Part print with two shaded views. Sizes in mm from the minimum x, y, z corner. Coordinates: 2 decimals unless noted, no trailing zeros. Order: outer loops, then holes, each group sorted by start corner. A loop starts at its lowest first (then second) coordinate and runs counter-clockwise, first axis right, second up. Notation, with made-up numbers: (-1, -37) - (54, -37) arc R17 ccw to (54, -21) - close; hole circle Ø3 at (56.25, 2.25). An arc over 180 degrees is marked (long way). Write each question's results on one line, items separated by ' | '. Start each with the question number.
Q1. Wall check: probe 1 along X at (y, z) = (51.5, 2.55) (1 decimal); probe 2 along Y at (x, z) = (7, 1.6); probe 3 along Y at (x, z) = (6, 2.4) (1 decimal). Give the ranges that are in metal, low to high.
Q2. Pin check, flat tips, straight feed: P1, Ø8, axis at x = 47, y = 39.5, coming from the -Z side; P2, Ø1.5, axis at y = 34.5, z = 2, coming from the +X side. Stop position of each tip, or through.
Q3. Band-saw the part on C-C, the plane x = 44.5. Write the cut outline in (y, z) (1 decimal).
Q4. Band-saw the part on A-A, the plane z = 1.6. Count the separate pieces of the cut face and the enclosed holes in it, then the cut area to 3 significant figures.
Q5. Band-saw the part on D-D, the plane y = 35.5. Write the cut outline in (x, z) (1 decimal), then the cut area to 3 significant figures.
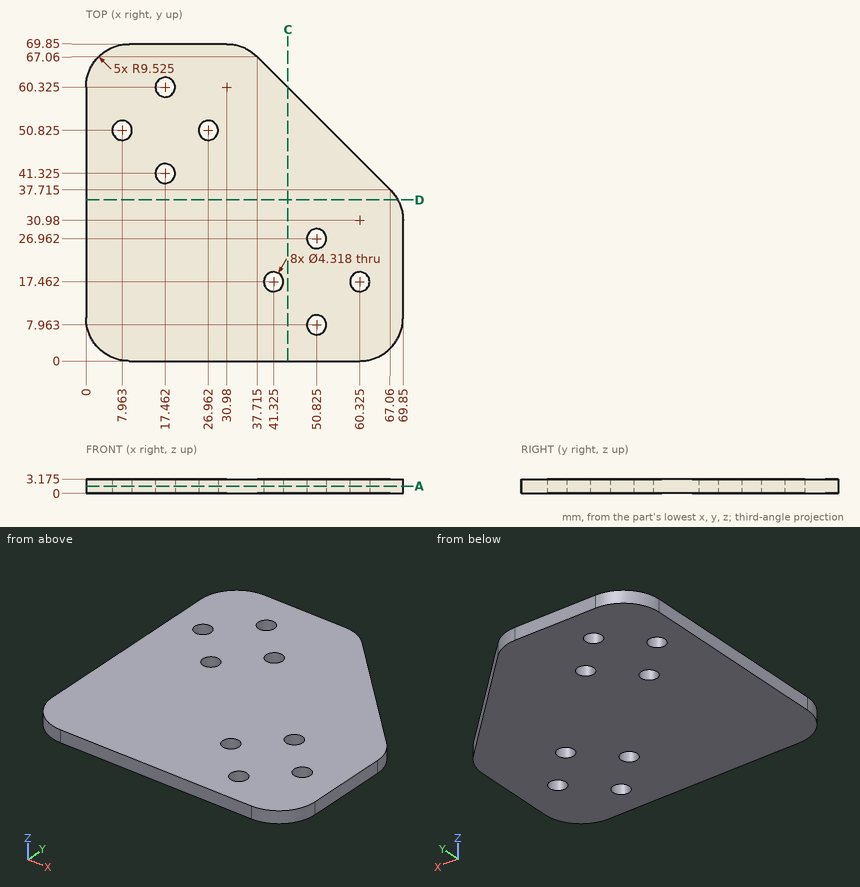
Results below:
1) probe 1: x = 0 to 5.9, 10 to 24.9, 29 to 53.3 | probe 2: y = 0.34 to 48.89, 52.76 to 69.51 | probe 3: y = 0.7 to 49.9, 51.7 to 69.2
2) P1: stops at z = 0 | P2: stops at x = 69.44
3) outline: (0, 0) - (60.3, 0) - (60.3, 3.2) - (0, 3.2) - close
4) separate pieces: 1 | enclosed holes: 8 | area: 4,090 mm²
5) outline: (0, 0) - (68.7, 0) - (68.7, 3.2) - (0, 3.2) - close | area: 218 mm²
